```python
from build123d import *

# Parameters (mm, degrees)
BOSS_EXTRUDE1_DEPTH = 3
CUT_EXTRUDE1_DEPTH  = 1
CUT_EXTRUDE2_REACH  = 136.027


with BuildPart() as part:
    # Sketch1 → Boss-Extrude1 (new body)
    with BuildSketch(Plane(origin=(0, 0, 0), x_dir=(1, 0, 0), z_dir=(0, 1, 0))):
        with BuildLine():
            Line((-5.431022837, 25.099874039), (-5.62533215, 25.099874039))
            ThreePointArc((-5.62533215, 25.099874039), (-7.746652493, 24.221194382), (-8.62533215, 22.099874039))
            Line((-8.62533215, 22.099874039), (-8.62533215, 14.358894177))
            Line((-8.62533215, 14.358894177), (131.37466785, 14.358894177))
            Line((131.37466785, 14.358894177), (131.37466785, 22.099874039))
            ThreePointArc((131.37466785, 22.099874039), (130.495988194, 24.221194382), (128.37466785, 25.099874039))
            Line((128.37466785, 25.099874039), (128.180358538, 25.099874039))
            ThreePointArc((128.180358538, 25.099874039), (126.694892152, 25.430743303), (125.49028015, 26.360794257))
            Line((125.49028015, 26.360794257), (-2.74094445, 26.360794257))
            ThreePointArc((-2.74094445, 26.360794257), (-3.945556452, 25.430743303), (-5.431022837, 25.099874039))
        make_face()
    extrude(amount=BOSS_EXTRUDE1_DEPTH)

    # Sketch2 → Cut-Extrude1 (cut)
    with BuildSketch(Plane.XZ):
        Polygon((5.157574014, -18.873414802), (5.80470943, -18.873414802), (5.80470943, -22.373414802), (5.490606866, -22.373414802), (5.490606866, -19.232389161), (4.952145328, -19.232389161), align=None)
    extrude(amount=-CUT_EXTRUDE1_DEPTH, mode=Mode.SUBTRACT)

    # Sketch3 → Cut-Extrude2 (cut, up to next)
    with BuildSketch(Plane(origin=(0, 3, 0), x_dir=(1, 0, 0), z_dir=(0, 1, 0)), mode=Mode.PRIVATE) as cut_extrude2_sk1:
        with BuildLine():
            ThreePointArc((41.109797099, 17.303114067), (42.709797099, 18.903114067), (41.109797099, 20.503114067))
            ThreePointArc((41.109797099, 20.503114067), (39.509797099, 18.903114067), (41.109797099, 17.303114067))
        make_face()
    cut_extrude2_tool1 = extrude(cut_extrude2_sk1.sketch, amount=-CUT_EXTRUDE2_REACH, mode=Mode.PRIVATE) & part.part
    # Sketch3 → Cut-Extrude2 (cut, up to next)
    with BuildSketch(Plane(origin=(0, 3, 0), x_dir=(1, 0, 0), z_dir=(0, 1, 0)), mode=Mode.PRIVATE) as cut_extrude2_sk2:
        with BuildLine():
            ThreePointArc((81.109797099, 17.303114067), (82.709797099, 18.903114067), (81.109797099, 20.503114067))
            ThreePointArc((81.109797099, 20.503114067), (79.509797099, 18.903114067), (81.109797099, 17.303114067))
        make_face()
    cut_extrude2_tool2 = extrude(cut_extrude2_sk2.sketch, amount=-CUT_EXTRUDE2_REACH, mode=Mode.PRIVATE) & part.part
    add(cut_extrude2_tool1.solids().sort_by_distance((41.109797, 3, -18.903114))[0], mode=Mode.SUBTRACT)
    add(cut_extrude2_tool2.solids().sort_by_distance((81.109797, 3, -18.903114))[0], mode=Mode.SUBTRACT)


solid = part.part
```
CAD build for the part. Positions are in the model's coordinates, mm. Coordinates: 2 decimals unless noted, no trailing zeros. Order: outer loops, then holes, each group sorted by start corner. A loop starts at its lowest first (then second) coordinate and runs counter-clockwise, first axis right, second up. Notation, with made-up numbers: M -5.75,15 L 31.25,15 A14 ccw 31.25,31 Z; hole C 84,21 d7. An arc over 180 degrees is marked long. Write each question's results on one line, items separated by ' | '. Start each with the question number.
Q1. Pull direction Z, two halves, no side cores. Call faces 1 (the cylindrical face through (81.039, 1.521, -17.305)), 2 (the cylindrical face through (-3.93, 1.48, -25.44)), 3 (the cylindrical face through (42.08, 1.52, -17.63)), 4 (the flat face through (131.375, 1, -18)): +Z half, -Z half, draft (parallel to the pull), parting line (faces both ways), or undercut.
Q2. Flat gauge pins, fed straight in: P1, Ø1, axis at x = 113.5, z = -25, coming from the -Y side; P2, Ø1, axis at y = 2.5, z = -24, coming from the -X side. Where does each tip first touch, or does it go through?
Q3. Cut at A-A (y = 2.1). List the corners of the cut face in (x, z).
Q4. Drill centre lines: probe 1 along X at (y, z) = (0.3, -21.5); probe 2 along X at (y, z) = (1.35, -18); probe 3 along X at (y, z) = (0.5, -18.25). Where is each one in solid material? Low to high. Write a range as from..to.
Found:
1) face 1: undercut | face 2: -Z half | face 3: undercut | face 4: draft
2) P1: y = 0 | P2: x = -8.28
3) outline: M -8.63,-22.1 A3 ccw -5.63,-25.1 L -5.43,-25.1 A3.5 cw -2.74,-26.36 L 125.49,-26.36 A3.5 cw 128.18,-25.1 L 128.37,-25.1 A3 ccw 131.37,-22.1 L 131.37,-14.36 L -8.63,-14.36 Z; hole C 41.11,-18.9 d3.2; hole C 81.11,-18.9 d3.2
4) probe 1: -8.63..5.49, 5.8..131.37 | probe 2: -8.63..39.79, 42.43..79.79, 82.43..131.37 | probe 3: -8.63..39.65, 42.57..79.65, 82.57..131.37
